Autodesk Inventor part; units mm, degrees
ref_plane "YZ Plane" through (0, 0, 0) normal (1, 0, 0) x (0, 1, 0)
ref_plane "XZ Plane" through (0, 0, 0) normal (0, 1, 0) x (-1, 0, 0)
ref_plane "XY Plane" through (0, 0, 0) normal (0, 0, 1) x (1, 0, 0)
sketch "Sketch1" plane through (0, 0, 0) normal (0, 1, 0) x (-1, 0, 0)
  line L0 (60, 50) -> (-60, 50)
  line L1 (-60, 50) -> (-60, -50)
  line L2 (-60, -50) -> (60, -50)
  line L3 (60, -50) -> (60, 50)
  line L4 (60, 50) -> (-60, -50) construction
  line L5 (-60, 50) -> (60, -50) construction
  point P0 (0, 0)
  dimension "d0" = 120
  dimension "d1" = 100
extrude "Extrusion1" add sketch "Sketch1" along normal blind 6
sketch "Sketch5" plane through (0, 6, 0) normal (0, 1, 0) x (1, 0, 0)
  circle A0 centre (-10.05, 0) radius 1.2295
  circle A1 centre (-10.05, 0) radius 10.4
  point P0 (0, 0)
  dimension "d16" = 20.8
extrude "Extrusion3" cut sketch "Sketch5" against normal blind 2.3 contours A0 | A1
hole "Hole1" at (-18.05, 6, -8.07) at (-18.05, 6, 8.07) at (-3.15, 6, 8) at (-3.15, 6, -8) at (10.07, 6, 7) at (17.37, 6, 0) at (10.07, 6, -7) direction (0, -1, 0) diameter 2.1 end through all
sketch "Sketch8" plane through (0, 6, 0) normal (0, 1, 0) x (1, 0, 0)
  arc A0 (-17.650182, -7.0991) -> (-17.08262, -7.661739) centre (-18.05, -8.07) ccw
  arc A1 (-17.08262, 7.661739) -> (-17.650182, 7.0991) centre (-18.05, 8.07) ccw
  arc A2 (-4.068914, -8.508032) -> (-2.512532, -7.165653) centre (-3.15, -8) ccw
  arc A3 (-2.512532, 7.165653) -> (-4.068914, 8.508032) centre (-3.15, 8) ccw
  circle A4 centre (10.07, -7) radius 1.05
  circle A5 centre (17.37, 0) radius 1.05
  circle A6 centre (10.07, 7) radius 1.05
  circle A7 centre (-18.05, -8.07) radius 2.05
  circle A8 centre (-18.05, 8.07) radius 2.05
  circle A9 centre (-3.15, -8) radius 2.05
  circle A10 centre (-3.15, 8) radius 2.05
  circle A11 centre (10.07, 7) radius 2.05
  circle A12 centre (10.07, -7) radius 2.05
  circle A13 centre (17.37, 0) radius 2.05
  point P0 (0, 0)
  dimension "d31" = 4.1
extrude "Extrusion6" cut sketch "Sketch8" against normal blind 3.5 contours A4 | A5 | A6 | A7 | A8 | A9 | A10 | A11 | A12 | A13
sketch "Sketch11" plane through (0, 6, 0) normal (0, 1, 0) x (1, 0, 0)
  circle A0 centre (-10.05, 0) radius 25
  circle A1 centre (-10.05, 0) radius 35
  circle A2 centre (-10.05, 0) radius 24.85
  circle A3 centre (-10.05, 0) radius 35.15
  point P0 (0, 0)
  dimension "d38" = 0.15
  dimension "d39" = 0.15
sketch "Sketch11 outline for Extrusion9" plane through (0, 6, 0) normal (0, 1, 0) x (1, 0, 0)
  circle A0 centre (-10.05, 0) radius 35.15
  circle A1 centre (-10.05, 0) radius 24.85
extrude "Extrusion9" cut sketch "Sketch11 outline for Extrusion9" against normal blind 2
sketch "Sketch12" plane through (0, 6, 0) normal (0, 1, 0) x (1, 0, 0)
  line L0 (-44.2, 50.07) -> (-44.2, -50.07) construction
  line L1 (-35.9, 50.07) -> (-35.9, -50.07) construction
  line L2 (35.9, 50.07) -> (35.9, -50.07) construction
  line L3 (44.2, 50.07) -> (44.2, -50.07) construction
  line L4 (60, 50) -> (-60, 50)
  line L5 (-40.05, -50.07) -> (-40.05, 50) construction
  line L6 (40.05, -50.07) -> (40.05, 50) construction
  line L7 (-44.2, -50.07) -> (-35.9, -50.07) construction
  line L8 (35.9, -50.07) -> (44.2, -50.07) construction
  line L9 (-60, 50) -> (-60, -50)
  line L10 (60, -50) -> (60, 50)
  line L11 (-60, 0) -> (60, 0) construction
  point P0 (0, 0)
  point P1 (-40.05, -38.07)
  point P2 (40.05, -38.07)
  point P3 (-40.05, 38.07)
  point P4 (40.05, 38.07)
  dimension "d42" = 12
hole "Hole2" at (-40.05, 6, 38.07) at (40.05, 6, 38.07) at (-40.05, 6, -38.07) at (40.05, 6, -38.07) direction (0, -1, 0) diameter 5.2 end through all counterbore diameter 10 counterbore depth 3
sketch "Sketch13" plane through (0, 0, 0) normal (0, -1, 0) x (1, 0, 0)
  circle A0 centre (-10.05, 0) radius 35.15
  line L0 (-19.05, 10.07) -> (19.05, 10.07)
  line L1 (20.05, 9.07) -> (20.05, -9.07)
  line L2 (19.05, -10.07) -> (-19.05, -10.07)
  line L3 (-20.05, -9.07) -> (-20.05, 9.07)
  arc A1 (-19.05, 10.07) -> (-20.05, 9.07) centre (-19.05, 9.07) ccw
  arc A2 (20.05, 9.07) -> (19.05, 10.07) centre (19.05, 9.07) ccw
  arc A3 (19.05, -10.07) -> (20.05, -9.07) centre (19.05, -9.07) ccw
  arc A4 (-20.05, -9.07) -> (-19.05, -10.07) centre (-19.05, -9.07) ccw
  point P0 (0, 0)
  point P1 (20.05, -10.07)
  point P2 (20.05, 10.07)
  point P3 (-20.05, -10.07)
  point P4 (-20.05, 0)
  dimension "d50" = 40.1
  dimension "d51" = 20.14
  dimension "d52" = 10
  dimension "d53" = 1
extrude "Extrusion10" cut sketch "Sketch13" against normal blind 0.5 contours L0 A2 L1 A3 L2 A4 L3 A1
sketch "Sketch14" plane through (0, 0.5, 0) normal (0, -1, 0) x (1, 0, 0)
  circle A0 centre (-10.05, 0) radius 24.85
  circle A1 centre (-10.05, 0) radius 6.5
  point P0 (0, 0)
  dimension "d56" = 13
extrude "Extrusion11" cut sketch "Sketch14" against normal through all contours A1
properties part number "axis_1_top_frame" material "Aluminum 6061-AHC"
Check sheet for the modelled part. Datum: model origin and axes. Units: mm. A direction names the side the tool comes from. Round coordinates to 2 decimals unless told otherwise and drop trailing zeros. Write each loop counter-clockwise with the first axis right and the second up, starting at its lowest first coordinate (ties: lowest second). Pieces come first, ordered by that corner, then holes. Notation, with made-up numbers: (33.25, -34.75) -> (68.25, -34.75) arc R29 cw to (68.25, -14.75) -> close; hole circle Ø7 at (-13.5, 38.5). An arc over 180 degrees is marked (long way). One line per question, with ' | ' between items. Start each with the question number.
1. Scan lines: line 1 along Z through (x, y) = (40.05, 1.85); line 2 along Z through (x, y) = (40.05, 4.8); line 3 along Z through (x, y) = (17.5, 1.8). Record each from-to range of solid material in increasing order. Write a range as from..to.
2. Depth check by flat-ended pin: pin 1 (6.5 mm diameter, centred on x = 10.07, z = 7, fed in from +Y); pin 2 (6 mm diameter, centred on x = 40.05, z = 38.07, fed in from +Y); pin 3 (3.5 mm diameter, centred on x = -3.15, z = -8, fed in from +Y); pin 4 (10 mm diameter, centred on x = 0, z = 1.5, fed in from -Y). Enter the tip coordinate at first touch or a pass-through.
3. Sectioned sample at B-B, the plane x = 40.05. Record the cut outline in (y, z), then the cut area to 3 significant figures.
4. Sectioned sample at C-C, the plane x = -10.05. Record the cut outline in (y, z).
5. Release check for a two-part mould opening along X. For faces 3 (the face through (1, 3, -50)), 4 (the face through (-38, 3, -36)) record: +X half, -X half, draft (parallel to the pull), parting line (faces both ways), or undercut.
6. Sectioned sample at D-D, the plane z = -15.5. Record the cut outline in (x, y).
7. Sectioned sample at A-A, the plane z = 38.07. Record the cut outline in (x, y), then the cut area to 3 significant figures.
8. Set-up check for faces 1 (the face through (-3.85, 2.08, 1.95)), 2 (the face through (16, 2.5, 0)): record each of +Z, -Z, +X, -X, +Y, -Y from which the full face is reachable in a straight line by a thin tool's end or side.
Taken from the geometry:
1) line 1: z = -50..-40.67, -35.47..35.47, 40.67..50 | line 2: z = -50..-43.07, -33.07..33.07, 43.07..50 | line 3: z = -50..-1.04, 1.04..50
2) pin 1: stops at y = 6 | pin 2: stops at y = 3 | pin 3: stops at y = 2.5 | pin 4: stops at y = 0.5
3) outline: (0, -50) -> (6, -50) -> (6, -43.07) -> (3, -43.07) -> (3, -40.67) -> (0, -40.67) -> close; (0, -35.47) -> (3, -35.47) -> (3, -33.07) -> (6, -33.07) -> (6, 33.07) -> (3, 33.07) -> (3, 35.47) -> (0, 35.47) -> close; (0, 40.67) -> (3, 40.67) -> (3, 43.07) -> (6, 43.07) -> (6, 50) -> (0, 50) -> close | area: 509 mm^2
4) outline: (0, -50) -> (6, -50) -> (6, -35.15) -> (4, -35.15) -> (4, -24.85) -> (6, -24.85) -> (6, -10.4) -> (3.7, -10.4) -> (3.7, -6.5) -> (0.5, -6.5) -> (0.5, -10.07) -> (0, -10.07) -> close; (0, 10.07) -> (0.5, 10.07) -> (0.5, 6.5) -> (3.7, 6.5) -> (3.7, 10.4) -> (6, 10.4) -> (6, 24.85) -> (4, 24.85) -> (4, 35.15) -> (6, 35.15) -> (6, 50) -> (0, 50) -> close
5) face 3: draft | face 4: undercut
6) outline: (-60, 0) -> (60, 0) -> (60, 6) -> (21.5, 6) -> (21.5, 4) -> (9.37, 4) -> (9.37, 6) -> (-29.47, 6) -> (-29.47, 4) -> (-41.6, 4) -> (-41.6, 6) -> (-60, 6) -> close
7) outline: (-60, 0) -> (-42.65, 0) -> (-42.65, 3) -> (-45.05, 3) -> (-45.05, 6) -> (-60, 6) -> close; (-37.45, 0) -> (37.45, 0) -> (37.45, 3) -> (35.05, 3) -> (35.05, 6) -> (-35.05, 6) -> (-35.05, 3) -> (-37.45, 3) -> close; (42.65, 0) -> (60, 0) -> (60, 6) -> (45.05, 6) -> (45.05, 3) -> (42.65, 3) -> close | area: 629 mm^2
8) face 1: +Y, -Y | face 2: +Y
